The model under review builds one solid part; all positions refer to its coordinate system, in mm. Face numbers are marked on the shaded views. Coordinates: 2 decimals unless noted, no trailing zeros. Write each loop counter-clockwise with the first axis right and the second up, starting at its lowest first coordinate (ties: lowest second). Pieces come first, ordered by that corner, then holes.
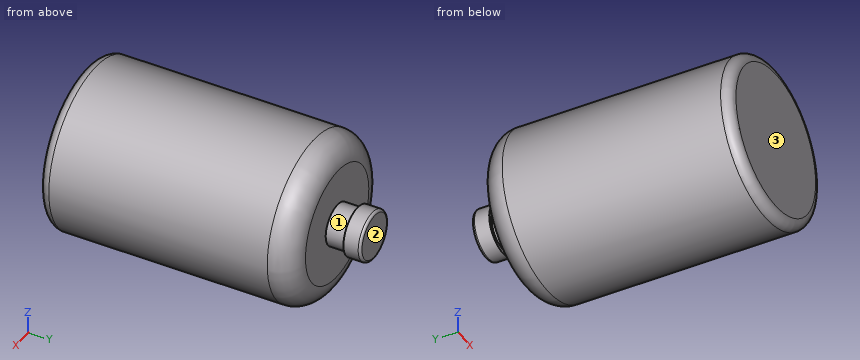
```python
from build123d import *

# Parameters (mm, degrees)
SKETCH1_R           = 33.25
BOSS_EXTRUDE1_DEPTH = 102.7
SKETCH2_R           = 10.05
BOSS_EXTRUDE2_DEPTH = 15.1
FILLET1_R           = 4
FILLET2_R           = 10
FILLET3_R           = 1
SKETCH4_R           = 10.05
SKETCH4_R_2         = 8.4
CUT_EXTRUDE1_DEPTH  = 8.1


with BuildPart() as part:
    # Sketch1 → Boss-Extrude1 (new body)
    with BuildSketch(Plane(origin=(0, 0, 0), x_dir=(1, 0, 0), z_dir=(0, 1, 0))):
        with Locations(Location((0, 0, 0), (0, 0, 270))):
            Circle(SKETCH1_R)
    extrude(amount=BOSS_EXTRUDE1_DEPTH)

    # Sketch2 → Boss-Extrude2 (add)
    with BuildSketch(Plane(origin=(0, 102.7, 0), x_dir=(1, 0, 0), z_dir=(0, 1, 0))):
        with Locations(Location((0, 0, 0), (0, 0, 270))):
            Circle(SKETCH2_R)
    extrude(amount=BOSS_EXTRUDE2_DEPTH)

    # Fillet1
    fillet1_edges = [part.edges().sort_by_distance(p)[0] for p in [
        (0, 0, -33.25),
    ]]
    fillet(fillet1_edges, radius=FILLET1_R)

    # Fillet2
    fillet2_edges = [part.edges().sort_by_distance(p)[0] for p in [
        (0, 102.7, -33.25),
    ]]
    fillet(fillet2_edges, radius=FILLET2_R)

    # Fillet3
    fillet3_edges = [part.edges().sort_by_distance(p)[0] for p in [
        (0, 117.8, -10.05),
    ]]
    fillet(fillet3_edges, radius=FILLET3_R)

    # Sketch4 → Cut-Extrude1 (cut)
    with BuildSketch(Plane(origin=(0, 102.7, 0), x_dir=(1, 0, 0), z_dir=(0, 1, 0))):
        with Locations(Location((0, 0, 0), (0, 0, 270))):
            Circle(SKETCH4_R)
        with Locations(Location((0, 0, 0), (0, 0, 270))):
            Circle(SKETCH4_R_2, mode=Mode.SUBTRACT)
    extrude(amount=CUT_EXTRUDE1_DEPTH, mode=Mode.SUBTRACT)


solid = part.part
```
Item 1: To check wall thickness, follow line 1 along Y through (x, z) = (-21, 0); line 2 along X through (y, z) = (69, -1); line 3 along Z through (x, y) = (3, 76.5). State the ranges of each line that lie inside material, in increasing order.
Solved:
line 1: y = 0 to 102.7
line 2: x = -33.23 to 33.23
line 3: z = -33.11 to 33.11
Item 2: Take a section at D-D, the plane y = 68.5. Write out the cut boundary in (x, z), plus the area to 3 significant figures.
Solved:
outline: circle Ø66.5 at (0, 0)
area: 3,470 mm2
Item 3: Take a section at C-C, the plane y = 109. Write out the cut boundary in (x, z), plus the area to 3 significant figures.
Solved:
outline: circle Ø16.8 at (0, 0)
area: 222 mm2
Item 4: Take a section at B-B, the plane z = 0. Write out the cut boundary in (x, y), plus the area to 3 significant figures.
Solved:
outline: (-33.25, 4) arc R4 ccw to (-29.25, 0) - (29.25, 0) arc R4 ccw to (33.25, 4) - (33.25, 92.7) arc R10 ccw to (23.25, 102.7) - (8.4, 102.7) - (8.4, 110.8) - (10.05, 110.8) - (10.05, 116.8) arc R1 ccw to (9.05, 117.8) - (-9.05, 117.8) arc R1 ccw to (-10.05, 116.8) - (-10.05, 110.8) - (-8.4, 110.8) - (-8.4, 102.7) - (-23.25, 102.7) arc R10 ccw to (-33.25, 92.7) - close
area: 7,060 mm2
Item 5: For pin 1 (3 mm diameter, centred on y = 31.5, z = 18, fed in from -X); pin 2 (5 mm diameter, centred on x = -8.5, z = 13.5, fed in from +Y); pin 3 (8 mm diameter, centred on y = 21.5, z = 10, fed in from +X), all flat-tipped, find the tip position at first contact; note any pin that passes through.
Solved:
pin 1: stops at x = -28.87
pin 2: stops at y = 102.7
pin 3: stops at x = 32.7
Item 6: Take a section at A-A, the plane x = 0. Write out the cut boundary in (y, z).
Solved:
outline: (0, -29.25) arc R4 ccw to (4, -33.25) - (92.7, -33.25) arc R10 ccw to (102.7, -23.25) - (102.7, -8.4) - (110.8, -8.4) - (110.8, -10.05) - (116.8, -10.05) arc R1 ccw to (117.8, -9.05) - (117.8, 9.05) arc R1 ccw to (116.8, 10.05) - (110.8, 10.05) - (110.8, 8.4) - (102.7, 8.4) - (102.7, 23.25) arc R10 ccw to (92.7, 33.25) - (4, 33.25) arc R4 ccw to (0, 29.25) - close
Item 7: Mouldability with a two-part tool opening along Y and no side actions: class the marked faces 1, 2 and 3 as pulls with the +Y half, pulls with the -Y half, needs draft (parallel to the pull), parting line crosses it, or undercut.
Solved:
face 1: undercut
face 2: pulls with the +Y half
face 3: pulls with the -Y half
